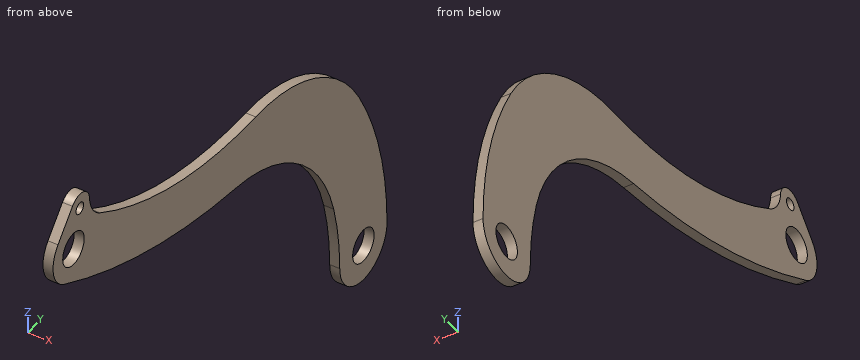
```python
from build123d import *

# Parameters (mm, degrees)
BOSS_EXTRUDE1_DEPTH = 1.5
SKETCH2_R           = 5
CUT_EXTRUDE1_DEPTH  = 142.810613143
SKETCH4_R           = 1.75
BOSS_EXTRUDE2_DEPTH = 3


with BuildPart() as part:
    # Sketch1 → Boss-Extrude1 (new, symmetric)
    with BuildSketch(Plane(origin=(0, 0, 0), x_dir=(0, 0, -1), z_dir=(1, 0, 0))):
        with BuildLine():
            ThreePointArc((0, 79), (11, 90), (0, 101))
            ThreePointArc((0, 101), (-25.350874614, 97.701945149), (-49.014054674, 88.027343403))
            ThreePointArc((-49.014054674, 88.027343403), (-68.978437503, 67.692387852), (-75.252234106, 39.89442974))
            ThreePointArc((-75.252234106, 39.89442974), (-79.876334442, -1.725579257), (-97.797422275, -39.573195612))
            ThreePointArc((-97.797422275, -39.573195612), (-94.917356951, -53.128320897), (-81.574017035, -49.387802533))
            ThreePointArc((-81.574017035, -49.387802533), (-66.010073659, -10.395208993), (-58.530464131, 30.917187762))
            ThreePointArc((-58.530464131, 30.917187762), (-46.946256543, 59.483246729), (-21.037120215, 76.184451628))
            ThreePointArc((-21.037120215, 76.184451628), (-10.612348227, 78.292988751), (0, 79))
        make_face()
    extrude(amount=BOSS_EXTRUDE1_DEPTH, both=True)

    # Sketch2 → Cut-Extrude1 (cut, through all)
    with BuildSketch(Plane(origin=(1.5, 0, 0), x_dir=(0, 0, -1), z_dir=(1, 0, 0))):
        with Locations((0, 90)):
            Circle(SKETCH2_R)
        with Locations((-90, -45)):
            Circle(SKETCH2_R)
    extrude(amount=-CUT_EXTRUDE1_DEPTH, mode=Mode.SUBTRACT)

    # Sketch4 → Boss-Extrude2 (add)
    with BuildSketch(Plane(origin=(1.5, 0, 0), x_dir=(0, 0, -1), z_dir=(1, 0, 0))):
        with BuildLine():
            Line((-104.046842635, -45.431522879), (-96.203913002, -52.194544007))
            ThreePointArc((-96.203913002, -52.194544007), (-96.739012984, -42.16802815), (-93.346869933, -32.717593358))
            ThreePointArc((-93.346869933, -32.717593358), (-96.754563068, -36.116875497), (-101.355592309, -37.530389374))
            ThreePointArc((-101.355592309, -37.530389374), (-105.36782436, -40.572667885), (-104.046842635, -45.431522879))
        make_face()
        with Locations((-101.108147002, -42.023580981)):
            Circle(SKETCH4_R, mode=Mode.SUBTRACT)
    extrude(amount=-BOSS_EXTRUDE2_DEPTH)


solid = part.part
```
The model under review builds one solid part; all positions refer to its coordinate system, in mm. Round coordinates to 2 decimals unless told otherwise and drop trailing zeros. Order: outer loops, then holes, each group sorted by start corner. A loop starts at its lowest first (then second) coordinate and runs counter-clockwise, first axis right, second up. Notation, with made-up numbers: (18.5, 69) -> (38.5, 69) arc R19 cw to (38.5, 94) -> close; hole circle Ø3 at (22, 73.5). An arc over 180 degrees is marked (long way). One line per item, written item: value. Start each with the question number.
Q1. Take a section at B-B (y = 90). Write out the cut boundary in (x, z), and give its area (3 significant figures).
Q2. Wall thickness on line 1 (Y direction, x = 0.8, z = 90); line 2 (Z direction, x = -0.65, y = 94); line 3 (Z direction, x = 0.8, y = 91): over which ranges is each line inside the solid? List them lowest first.
Q3. Take a section at D-D (y = 15). Write out the cut boundary in (x, z).
Q4. Take a section at C-C (x = -0.15). Write out the cut boundary in (y, z).
Q5. Take a section at A-A (z = -2). Write out the cut boundary in (x, y).
Q6. Clearance check with flat-ended pins moving along their axes: pin 1 Ø1.5 at (x, y) = (0, 27.5) entering from -Z; pin 2 Ø11.5 at (y, z) = (90, 0) entering from -X; pin 3 Ø1.5 at (x, z) = (-0.5, 84) entering from -Y; pin 4 Ø3 at (y, z) = (-42.02, 101.11) entering from +X. State where each tip first meets the part, or that it passes through.
Reported:
1. outline: (-1.5, -11) -> (1.5, -11) -> (1.5, -5) -> (-1.5, -5) -> close; (-1.5, 5) -> (1.5, 5) -> (1.5, 45.37) -> (-1.5, 45.37) -> close
1. area: 139 mm2
2. line 1: y = -54.5 to -50, -40 to -26.83
2. line 2: z = -10.25 to -3, 3 to 36.58
2. line 3: z = -10.95 to -4.9, 4.9 to 43.38
3. outline: (-1.5, 60.4) -> (1.5, 60.4) -> (1.5, 76.33) -> (-1.5, 76.33) -> close
4. outline: (-52.19, 96.2) arc R9.5 ccw to (-49.39, 81.57) arc R209.58 ccw to (30.92, 58.53) arc R51.09 cw to (76.18, 21.04) arc R80 cw to (79, 0) arc R11 ccw to (101, 0) arc R99.08 ccw to (88.03, 49.01) arc R52.08 ccw to (39.89, 75.25) arc R126.87 cw to (-32.72, 93.35) arc R10 cw to (-37.53, 101.36) arc R4.5 ccw to (-45.43, 104.05) -> close; hole circle Ø10 at (-45, 90); hole circle Ø3.5 at (-42.02, 101.11); hole circle Ø10 at (90, 0)
5. outline: (-1.5, 79.18) -> (1.5, 79.18) -> (1.5, 85.42) -> (-1.5, 85.42) -> close; (-1.5, 94.58) -> (1.5, 94.58) -> (1.5, 100.82) -> (-1.5, 100.82) -> close
6. pin 1: stops at z = 58.76
6. pin 2: stops at x = -1.5
6. pin 3: stops at y = -52.92
6. pin 4: passes through
